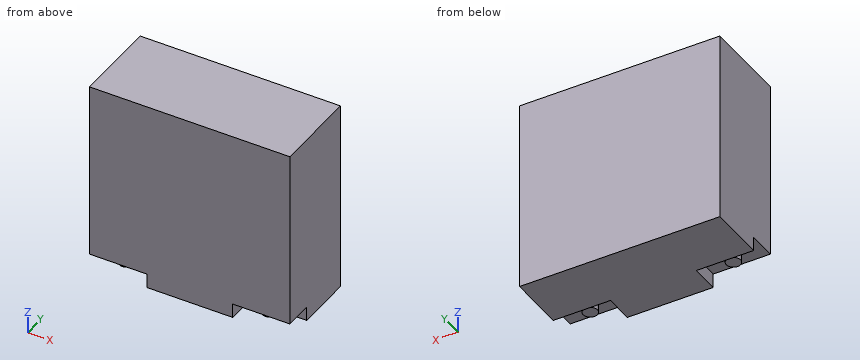
from build123d import *

# Parameters (mm, degrees)
SKETCH1_W           = 177.8
SKETCH1_H           = 76.2
BOSS_EXTRUDE1_DEPTH = 171.45
SKETCH2_W           = 50.8
SKETCH2_H           = 25.4
CUT_EXTRUDE1_DEPTH  = 12.7
SKETCH3_R           = 6.35
BOSS_EXTRUDE2_DEPTH = 6.35


with BuildPart() as part:
    # Sketch1 → Boss-Extrude1 (new body)
    with BuildSketch(Plane.XY):
        Rectangle(SKETCH1_W, SKETCH1_H)
    extrude(amount=BOSS_EXTRUDE1_DEPTH)

    # Sketch2 → Cut-Extrude1 (cut)
    with BuildSketch(Plane(origin=(0, 0, 0), x_dir=(-1, 0, 0), z_dir=(0, 0, -1))):
        with Locations((-63.5, -25.4)):
            Rectangle(SKETCH2_W, SKETCH2_H)
        with Locations((63.5, -25.4)):
            Rectangle(SKETCH2_W, SKETCH2_H)
    extrude(amount=-CUT_EXTRUDE1_DEPTH, mode=Mode.SUBTRACT)

    # Sketch3 → Boss-Extrude2 (add)
    with BuildSketch(Plane(origin=(0, 0, 12.7), x_dir=(-1, 0, 0), z_dir=(0, 0, -1))):
        with Locations(Location((-63.5, -25.4, 0), (0, 0, 180))):
            Circle(SKETCH3_R)
        with Locations(Location((63.5, -25.4, 0), (0, 0, 180))):
            Circle(SKETCH3_R)
    extrude(amount=BOSS_EXTRUDE2_DEPTH)


solid = part.part
Verification items for the finished model (mm, model axes). Coordinates: 2 decimals unless noted, no trailing zeros. Write each loop counter-clockwise with the first axis right and the second up, starting at its lowest first coordinate (ties: lowest second). Pieces come first, ordered by that corner, then holes. Notation, with made-up numbers: (12.5, 49) -> (66.5, 49) arc R14 ccw to (66.5, 61) -> close; hole circle Ø11 at (79.5, 53). An arc over 180 degrees is marked (long way). One line per item, written item: value. Start each with the question number.
Q1. Cross-section at B-B on x = -49. Enter the section's corners in (y, z), and give its area (3 significant figures).
Q2. Go/stop test with flat-tipped pins: P1, Ø6.5, axis at x = 66, y = -27, coming from the -Z side; P2, Ø14, axis at x = -60, z = 5.5, coming from the -Y side; P3, Ø10, axis at x = 55.5, z = 6, coming from the -Y side. Record where each tip stops, or that it passes through.
Q3. Cross-section at A-A on y = -25.4. Enter the section's corners in (x, z), and give its area (3 significant figures).
Q4. Cross-section at C-C on x = 63.5. Enter the section's corners in (y, z), and give its area (3 significant figures).
Q5. Thickness scan on L1, parallel to Z at x = -77.5, y = -28.5; L2, parallel to Z at x = 65.5, y = -23.5; L3, parallel to Y at x = -73, z = 12.5. Record the ranges inside material, lowest first. Write a range as from..to.
Checked values:
1. outline: (-38.1, 12.7) -> (-12.7, 12.7) -> (-12.7, 0) -> (38.1, 0) -> (38.1, 171.45) -> (-38.1, 171.45) -> close
1. area: 12,700 mm²
2. P1: stops at z = 6.35
2. P2: stops at y = -31.75
2. P3: stops at y = -30.99
3. outline: (-88.9, 12.7) -> (-69.85, 12.7) -> (-69.85, 6.35) -> (-57.15, 6.35) -> (-57.15, 12.7) -> (-38.1, 12.7) -> (-38.1, 0) -> (38.1, 0) -> (38.1, 12.7) -> (57.15, 12.7) -> (57.15, 6.35) -> (69.85, 6.35) -> (69.85, 12.7) -> (88.9, 12.7) -> (88.9, 171.45) -> (-88.9, 171.45) -> close
3. area: 29,400 mm²
4. outline: (-38.1, 12.7) -> (-31.75, 12.7) -> (-31.75, 6.35) -> (-19.05, 6.35) -> (-19.05, 12.7) -> (-12.7, 12.7) -> (-12.7, 0) -> (38.1, 0) -> (38.1, 171.45) -> (-38.1, 171.45) -> close
4. area: 12,800 mm²
5. L1: z = 12.7..171.45
5. L2: z = 6.35..171.45
5. L3: y = -12.7..38.1
